Build history of the part. All positions in model axes, mm. Face numbers are marked on the shaded views. A direction names the side the tool comes from. Round coordinates to 2 decimals unless told otherwise and drop trailing zeros. Order: outer loops, then holes, each group sorted by start corner. A loop starts at its lowest first (then second) coordinate and runs counter-clockwise, first axis right, second up. Notation, with made-up numbers: (57.5, 10.25) -> (113.5, 10.25) arc R20 ccw to (113.5, 25.25) -> close; hole circle Ø7 at (44, -37). An arc over 180 degrees is marked (long way). Write item = value, one per line.
from build123d import *

# Parameters (mm, degrees)
BOSS_EXTRUDE1_DEPTH = 30
SHELL1_T            = -3
SKETCH2_R           = 1.75
CUT_EXTRUDE1_DEPTH  = 10


with BuildPart() as part:
    # Sketch1 → Boss-Extrude1 (new body)
    with BuildSketch(Plane(origin=(0, 0, 0), x_dir=(1, 0, 0), z_dir=(0, 1, 0))):
        Polygon((0, 0), (80, 0), (0, 100), align=None)
    extrude(amount=BOSS_EXTRUDE1_DEPTH)

    # Shell1
    shell1_openings = [part.faces().sort_by_distance(p)[0] for p in [
        (40, 15, -50),
    ]]
    offset(amount=SHELL1_T, openings=shell1_openings, kind=Kind.INTERSECTION)

    # Sketch2 → Cut-Extrude1 (cut)
    with BuildSketch(Plane.ZY):
        with Locations((-15, 15)):
            Circle(SKETCH2_R)
        with Locations((-40, 15)):
            Circle(SKETCH2_R)
        with Locations((-65, 15)):
            Circle(SKETCH2_R)
        with Locations((-90, 15)):
            Circle(SKETCH2_R)
    extrude(amount=-CUT_EXTRUDE1_DEPTH, mode=Mode.SUBTRACT)


solid = part.part
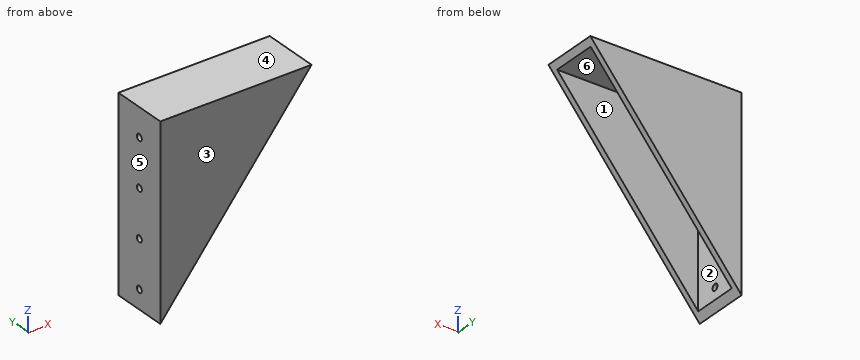
Q1. Mould opens along Y. For the marked faces 1, 2, 3 and 4 say: released by +Y, released by -Y, zero draft, split by the parting line, or undercut.
Check values:
face_1 = undercut
face_2 = undercut
face_3 = released by -Y
face_4 = zero draft
Q2. Cut at C-C, the plane x = 10. List the corners of the cut face in (y, z).
Check values:
outline = (0, -87.5) -> (3, -87.5) -> (3, -3) -> (27, -3) -> (27, -87.5) -> (30, -87.5) -> (30, 0) -> (0, 0) -> close
Q3. Probe probe 1 along Y at (x, z) = (14, -33.5); probe 2 along X at (y, z) = (5.75, -35); probe 3 along Z at (x, y) = (41, 9.5). List the from-to ranges inside material, lowest first.
Check values:
probe_1 = 0 to 3, 27 to 30
probe_2 = 0 to 3
probe_3 = -3 to 0
Q4. Cut at B-B, the plane z = -40. List the corners of the cut face in (x, y), and give its area (4 significant figures).
Check values:
outline = (0, 0) -> (48, 0) -> (48, 3) -> (3, 3) -> (3, 13.25) -> (0, 13.25) -> close; (0, 16.75) -> (3, 16.75) -> (3, 27) -> (48, 27) -> (48, 30) -> (0, 30) -> close
area = 349.5 mm²
Q5. Cut at A-A, the plane y = 15. List the corners of the cut face in (x, z).
Check values:
outline = (0, -100) -> (3, -96.25) -> (3, -91.75) -> (0, -91.75) -> close; (0, -88.25) -> (3, -88.25) -> (3, -66.75) -> (0, -66.75) -> close; (0, -63.25) -> (3, -63.25) -> (3, -41.75) -> (0, -41.75) -> close; (0, -38.25) -> (3, -38.25) -> (3, -16.75) -> (0, -16.75) -> close; (0, -13.25) -> (3, -13.25) -> (3, -3) -> (77.6, -3) -> (80, 0) -> (0, 0) -> close
Q6. Which spindle directions (+Z, -Z, +X, -X, +Y, -Y) get a long thin tool onto all of the face, cutting with end or side? Do the marked faces 5 and 6. Say none if no direction does.
Check values:
face_5 = +Z, -Z, -X, +Y, -Y
face_6 = -Z, +X
Q7. Flat gauge pin, fed straight in: pin 1 (1.5 mm diameter, centred on x = 45.5, y = 19.5, fed in from -Z). Where does the tip first touch, or does it go through?
Check values:
pin_1 = -3
Q8. Cut at D-D, the plane z = -82. List the corners of the cut face in (x, y).
Check values:
outline = (0, 0) -> (14.4, 0) -> (14.4, 3) -> (3, 3) -> (3, 27) -> (14.4, 27) -> (14.4, 30) -> (0, 30) -> close
